Autodesk Inventor part; units mm, degrees
ref_plane "Work Plane1" through (-21, -21, -14) normal (0, 0, 1) x (1, 0, 0)
ref_plane "Work Plane2" through (-21.15, 33.85, -45.625) normal (0, 1, 0) x (0, 0, 1)
ref_plane "YZ Plane" through (0, 0, 0) normal (1, 0, 0) x (0, 1, 0)
sketch "Sketch1" plane through (0, 0, 0) normal (0, 0, 1) x (1, 0, 0)
  line L0 (-20, 16.5858) -> (-16.5858, 20)
  line L1 (-20, -16.5858) -> (-20, 16.5858)
  line L2 (-16.5858, -20) -> (-20, -16.5858)
  line L3 (16.5858, -20) -> (-16.5858, -20)
  line L4 (20, -16.5858) -> (16.5858, -20)
  line L5 (20, 16.5858) -> (20, -16.5858)
  line L6 (16.5858, 20) -> (20, 16.5858)
  line L7 (-16.5858, 20) -> (16.5858, 20)
  circle A0 centre (15.5, -15.5) radius 1.5
  circle A1 centre (-15.5, 15.5) radius 1.5
  circle A2 centre (-15.5, -15.5) radius 1.5
  circle A3 centre (15.5, 15.5) radius 1.5
  circle A4 centre (0, 0) radius 11
  circle A5 centre (0, 0) radius 4.9
  line L8 (13.1931, -21.15) -> (-13.1931, -21.15)
  line L9 (-21.15, -13.1931) -> (-21.15, 13.1931)
  line L10 (21.15, 21.15) -> (-21.15, 21.15)
  line L11 (-21.15, 21.15) -> (-21.15, -21.15)
  line L12 (-21.15, -21.15) -> (21.15, -21.15)
  line L13 (21.15, -21.15) -> (21.15, 21.15)
  line L14 (21.15, 21.15) -> (-21.15, -21.15) construction
  line L15 (-21.15, 21.15) -> (21.15, -21.15) construction
  line L16 (23.15, -23.15) -> (-23.15, -23.15)
  line L17 (-23.15, -23.15) -> (-23.15, 21.15)
  line L18 (23.15, 21.15) -> (23.15, -23.15)
  line L19 (23.15, 21.15) -> (-23.15, 21.15)
  line L20 (-23.15, 21.15) -> (-23.1187, 21.15)
  line L21 (23.15, 21.15) -> (21.15, 21.15)
  line L22 (-13.1931, -21.15) -> (13.1931, -21.15)
  dimension "d0" = 2
extrude "Extrusion1" add sketch "Sketch1" along normal blind 2 contours L0 L7 L6 L5 L4 L3 L2 L1 | L12 L13 L19 L18 L16 L17 L11 L9 L8 | L8 L12 L11 L9 L10 L13
sketch "Sketch2" plane through (0, 0, 0) normal (0, 0, -1) x (-1, 0, 0)
  line L0 (21, -10) -> (21, 10)
  line L1 (-21, 10) -> (-21, -10)
  line L2 (-198.65, 21.15) -> (16.15, 21.15)
  line L3 (21, -21.15) -> (-21, -21.15)
  line L4 (-21, -21.15) -> (-21, 21.15)
  line L5 (-21, 21.15) -> (21, 21.15)
  line L6 (21, 21.15) -> (21, -21.15)
  line L7 (21, -21.15) -> (-21, 21.15) construction
  line L8 (-21, -21.15) -> (21, 21.15) construction
  line L9 (23.15, -23.15) -> (-23.15, -23.15)
  line L10 (-23.15, -23.15) -> (-23.15, 21.15)
  line L11 (23.15, 21.15) -> (23.15, -23.15)
  line L12 (-23.15, 21.15) -> (23.15, 21.15)
  line L13 (21, 21.15) -> (23.15, 21.15)
  line L14 (23.15, 21.15) -> (-21, 21.15)
  line L15 (-21, 21.15) -> (-23.15, 21.15)
  point P0 (0, 0)
ref_plane "Work Plane1" through (-21, -21, -14) normal (0, 0, 1) x (1, 0, 0)
extrude "Extrusion2" add sketch "Sketch2" along normal up to surface (14 mm away) contours L0 L6 L12 L11 L9 L10 L2 L4 L1 L3
sketch "Sketch3" plane through (-23.15, 21.15, 2) normal (0, 1, 0) x (1, 0, 0)
  line L0 (44.15, 2) -> (2.15, 2)
  line L1 (2.15, 2) -> (2.15, 16)
  line L2 (0, 16) -> (2.15, 16)
  line L3 (0, 16) -> (0, 0)
  line L4 (46.3, 0) -> (0, 0)
  line L5 (46.3, 0) -> (46.3, 16)
  line L6 (44.15, 16) -> (46.3, 16)
  line L7 (44.15, 2) -> (44.15, 16)
  arc A0 (2, -201.375) -> (7, -206.375) centre (7, -201.375) ccw
  line L8 (7, -206.375) -> (221.8, -206.375)
  arc A1 (221.8, -206.375) -> (226.8, -201.375) centre (221.8, -201.375) ccw
  line L9 (226.8, -201.375) -> (226.8, -174.375)
  arc A2 (226.8, -174.375) -> (221.8, -169.375) centre (221.8, -174.375) ccw
  line L10 (221.8, -169.375) -> (151.8, -169.375)
  arc A3 (146.8, -164.375) -> (151.8, -169.375) centre (151.8, -164.375) ccw
  line L11 (146.8, -164.375) -> (146.8, 5.625)
  arc A4 (151.8, 10.625) -> (146.8, 5.625) centre (151.8, 5.625) ccw
  line L12 (151.8, 10.625) -> (221.8, 10.625)
  arc A5 (221.8, 10.625) -> (226.8, 15.625) centre (221.8, 15.625) ccw
  line L13 (226.8, 15.625) -> (226.8, 42.625)
  arc A6 (226.8, 42.625) -> (221.8, 47.625) centre (221.8, 42.625) ccw
  line L14 (221.8, 47.625) -> (7, 47.625)
  arc A7 (7, 47.625) -> (2, 42.625) centre (7, 42.625) ccw
  line L15 (2, 42.625) -> (2, 5)
  arc A8 (2, 5) -> (7, 0) centre (7, 5) ccw
  line L16 (7, 0) -> (101.6, 0)
  line L17 (101.6, -158.75) -> (7, -158.75)
  arc A9 (7, -158.75) -> (2, -163.75) centre (7, -163.75) ccw
  line L18 (2, -163.75) -> (2, -201.375)
  line L19 (2, 5) -> (0, 5)
  circle A10 centre (208.3, 29.125) radius 5
  circle A11 centre (208.3, -187.875) radius 5
  circle A12 centre (20.5, 29.125) radius 5
  circle A13 centre (20.5, -187.875) radius 5
  arc A14 (103.6, -2) -> (101.6, 0) centre (101.6, -2) ccw
  line L20 (103.6, -2) -> (103.6, -156.75)
  arc A15 (101.6, -158.75) -> (103.6, -156.75) centre (101.6, -156.75) ccw
  point P0 (23.15, 2)
  point P1 (2, 16)
ref_plane "Work Plane2" through (-21.15, 33.85, -45.625) normal (0, 1, 0) x (0, 0, 1)
extrude "Extrusion3" add sketch "Sketch3" along normal up to surface (12.7 mm away) contours A8 L4 L3 L19 L1 L0 | L0 L1 A8 | L19 L3 L2 L15
sketch "Sketch4" plane through (-23.15, -23.15, -14) normal (-1, 0, 0) x (0, 0, 1)
  line L0 (0, 0) -> (0, 57)
  line L1 (16, 0) -> (16, 57)
  line L2 (0, 57) -> (16, 57)
  line L3 (16, 57) -> (16, 44.5)
  line L4 (16, 44.5) -> (0, 44.5)
  line L5 (0, 44.5) -> (0, 57)
  circle A0 centre (8, 50.75) radius 2.5
  point P0 (14, 23.15)
  dimension "d7" = 12.5
  dimension "d8" = 5
extrude "Extrusion4" cut sketch "Sketch4" against normal blind 2 contours A0
ref_plane "Work Plane3" through (81.25, 21.15, 81.375) normal (0, -1, 0) x (0, 0, 1)
sketch "Sketch5" plane through (81.25, 21.15, 81.375) normal (0, -1, 0) x (0, 0, 1)
  line L0 (-95.375, 58.1) -> (-79.375, 58.1)
  line L1 (-95.375, 58.1) -> (-79.375, 58.1)
  line L2 (-79.375, 104.4) -> (-79.375, 58.1)
  line L3 (-95.375, 104.4) -> (-79.375, 104.4)
  line L4 (-95.375, 58.1) -> (-95.375, 104.4)
  line L5 (-95.375, 58.1) -> (-79.375, 58.1)
  line L6 (-79.375, 58.1) -> (-79.375, 42.1)
  line L7 (-79.375, 42.1) -> (-95.375, 42.1)
  line L8 (-95.375, 42.1) -> (-95.375, 58.1)
  circle A0 centre (-87.375, 50.1) radius 2.5
  point P0 (-81.375, 81.25)
  dimension "d11" = 16
  dimension "d12" = 16
  dimension "d13" = 5
extrude "Extrusion6" add sketch "Sketch5" along normal blind 5 contours L0 L6 L7 L8
properties part number "PancakeNema17MotorMount"
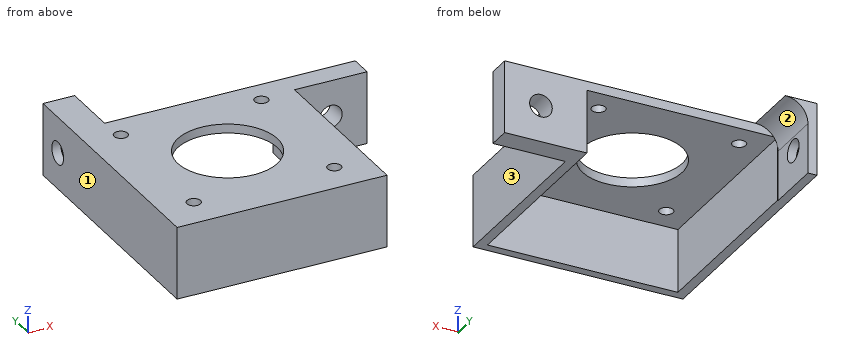
Geometry check sheet. Reference: the model listing, model coordinates, mm. Face numbers are marked on the shaded views. A direction names the side the tool comes from. Round coordinates to 2 decimals unless told otherwise and drop trailing zeros. Order: outer loops, then holes, each group sorted by start corner. A loop starts at its lowest first (then second) coordinate and runs counter-clockwise, first axis right, second up. Notation, with made-up numbers: M 34.25,34.5 L 45.25,34.5 A16 ccw 45.25,50.5 Z; hole C -33.75,-28 d11. An arc over 180 degrees is marked long. Answer as CSV lines item,"result".
1) Tool access check on the marked faces 1, 2 and 3. Record the directions out of +Z, -Z, +X, -X, +Y, -Y that give a thin tool (end or side, any length) a straight path to the whole face; none if there is none.
Entries:
face 1,"+Z, -Z, -X, +Y, -Y"
face 2,"-Z, +X, +Y"
face 3,"+Z, -Z, +X, -Y"
2) Gauge pin test, flat ends, axial feed: pin 1 Ø3.5 at (x, y) = (-15.5, 15.5) entering from +Z; pin 2 Ø5 at (y, z) = (4, -4) entering from +X; pin 3 Ø2.5 at (x, y) = (15.5, -15.5) entering from +Z; pin 4 Ø1 at (x, y) = (-3, -15.5) entering from -Z. Record the tip position at first contact, or that the pin passes through.
Entries:
pin 1,"z = 2"
pin 2,"x = 23.15"
pin 3,"through"
pin 4,"z = 0"
3) Sectioned sample at D-D on z = -13. Record the cut outline in (x, y).
Entries:
outline,"M -23.15,-23.15 L 23.15,-23.15 L 23.15,16.15 L 39.15,16.15 L 39.15,21.15 L 21,21.15 L 21,-21.15 L -21,-21.15 L -21,21.15 L -21.15,21.15 L -21.15,33.85 L -23.15,33.85 Z"
4) Sectioned sample at B-B on x = 0. Record the cut outline in (y, z), and give its area (3 significant figures).
Entries:
outline,"M -23.15,-14 L -21.15,-14 L -21.15,0 L -11,0 L -11,2 L -23.15,2 Z; M 11,0 L 21.15,0 L 21.15,2 L 11,2 Z"
area,"72.6 mm2"
5) Sectioned sample at A-A on y = 27.6. Record the cut outline in (x, z), and give its area (3 significant figures).
Entries:
outline,"M -23.15,-14 L -21.15,-14 L -21.15,-8.5 L -23.15,-8.5 Z; M -23.15,-3.5 L -21.15,-3.5 L -21.15,-3 A5 cw -16.15,2 L -23.15,2 Z"
area,"27.4 mm2"
6) Sectioned sample at C-C on x = 15.5. Record the cut outline in (y, z), and give its area (3 significant figures).
Entries:
outline,"M -23.15,-14 L -21.15,-14 L -21.15,0 L -17,0 L -17,2 L -23.15,2 Z; M -14,0 L 14,0 L 14,2 L -14,2 Z; M 17,0 L 21.15,0 L 21.15,2 L 17,2 Z"
area,"105 mm2"
7) Thickness scan on probe 1 along Y at (x, z) = (-15.5, 1); probe 2 along X at (y, z) = (19.35, -6); probe 3 along X at (y, z) = (12.5, -8.75). Record the ranges inside material, lowest first. Write a range as [from, to].
Entries:
probe 1,"[-23.15, -17], [-14, 14], [17, 21.15]"
probe 2,"[-23.15, -21], [21, 28.65], [33.65, 39.15]"
probe 3,"[-23.15, -21], [21, 23.15]"
